Check sheet for the modelled part. Datum: model origin and axes. Units: mm. Round coordinates to 2 decimals unless told otherwise and drop trailing zeros. Order: outer loops, then holes, each group sorted by start corner. A loop starts at its lowest first (then second) coordinate and runs counter-clockwise, first axis right, second up. Notation, with made-up numbers: (12, 82) -> (61, 82) arc R13 ccw to (61, 101) -> close; hole circle Ø7 at (14, -7.5). An arc over 180 degrees is marked (long way). Answer in a Markdown table with one row per item.
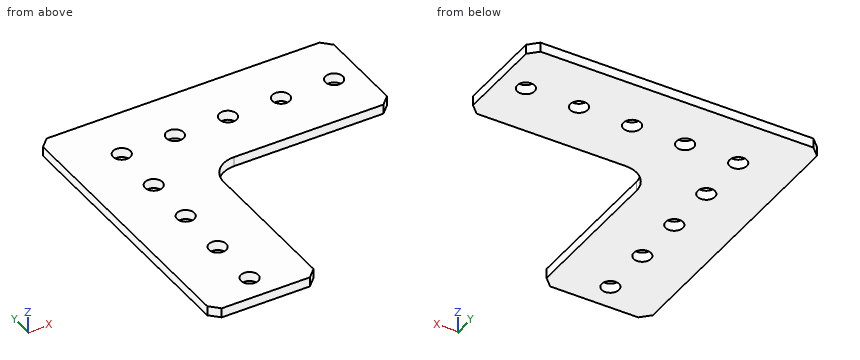
```python
from build123d import *

# Parameters (mm, degrees)
SKETCH1_R           = 2.0701
BOSS_EXTRUDE1_DEPTH = 2.286


with BuildPart() as part:
    # Sketch1 → Boss-Extrude1 (new body)
    with BuildSketch(Plane(origin=(0, 0, 0), x_dir=(-1, 0, 0), z_dir=(0, 0, -1))):
        with BuildLine():
            Line((10.414, 12.573), (-54.864, 12.573))
            Line((-54.864, 12.573), (-57.023, 10.414))
            Line((-57.023, 10.414), (-57.023, -10.668))
            Line((-57.023, -10.668), (-54.864, -12.827))
            Line((-54.864, -12.827), (-19.177, -12.827))
            ThreePointArc((-19.177, -12.827), (-14.686871939, -14.686871939), (-12.827, -19.177))
            Line((-12.827, -19.177), (-12.827, -54.864))
            Line((-12.827, -54.864), (-10.668, -57.023))
            Line((-10.668, -57.023), (10.414, -57.023))
            Line((10.414, -57.023), (12.573, -54.864))
            Line((12.573, -54.864), (12.573, 10.414))
            Line((12.573, 10.414), (10.414, 12.573))
        make_face()
        with Locations((0, -50.8)):
            Circle(SKETCH1_R, mode=Mode.SUBTRACT)
        with Locations((0, -25.4)):
            Circle(SKETCH1_R, mode=Mode.SUBTRACT)
        with Locations((-38.1, 0)):
            Circle(SKETCH1_R, mode=Mode.SUBTRACT)
        with Locations((-12.7, 0)):
            Circle(SKETCH1_R, mode=Mode.SUBTRACT)
        Circle(SKETCH1_R, mode=Mode.SUBTRACT)
        with Locations((-25.4, 0)):
            Circle(SKETCH1_R, mode=Mode.SUBTRACT)
        with Locations((0, -12.7)):
            Circle(SKETCH1_R, mode=Mode.SUBTRACT)
        with Locations((0, -38.1)):
            Circle(SKETCH1_R, mode=Mode.SUBTRACT)
        with Locations((-50.8, 0)):
            Circle(SKETCH1_R, mode=Mode.SUBTRACT)
    extrude(amount=-BOSS_EXTRUDE1_DEPTH)


solid = part.part
```
(1) Section check C-C on y = 0. Record the boundary of the cut face in (x, z), plus the area to 3 significant figures.
Solutions:
| item | result |
|---|---|
| outline | (-12.57, 0) -> (-2.07, 0) -> (-2.07, 2.29) -> (-12.57, 2.29) -> close; (2.07, 0) -> (10.63, 0) -> (10.63, 2.29) -> (2.07, 2.29) -> close; (14.77, 0) -> (23.33, 0) -> (23.33, 2.29) -> (14.77, 2.29) -> close; (27.47, 0) -> (36.03, 0) -> (36.03, 2.29) -> (27.47, 2.29) -> close; (40.17, 0) -> (48.73, 0) -> (48.73, 2.29) -> (40.17, 2.29) -> close; (52.87, 0) -> (57.02, 0) -> (57.02, 2.29) -> (52.87, 2.29) -> close |
| area | 112 mm^2 |
(2) Scan lines: probe 1 along Y at (x, z) = (0, 1.75); probe 2 along Y at (x, z) = (38.1, 1); probe 3 along X at (y, z) = (-27.5, 0.2). Record each from-to range of solid material in increasing order. Write a range as from..to.
Solutions:
| item | result |
|---|---|
| probe 1 | -57.02..-52.87, -48.73..-40.17, -36.03..-27.47, -23.33..-14.77, -10.63..-2.07, 2.07..12.57 |
| probe 2 | -12.83..-2.07, 2.07..12.57 |
| probe 3 | -12.57..12.83 |
(3) Section check A-A on x = 25.4. Record the boundary of the cut face in (y, z).
Solutions:
| item | result |
|---|---|
| outline | (-12.83, 0) -> (-2.07, 0) -> (-2.07, 2.29) -> (-12.83, 2.29) -> close; (2.07, 0) -> (12.57, 0) -> (12.57, 2.29) -> (2.07, 2.29) -> close |
(4) Depth check by flat-ended pin: pin 1 Ø1 at (x, z) = (41.5, 0.5) entering from -Y. Enter the tip coordinate at first touch or a pass-through.
Solutions:
| item | result |
|---|---|
| pin 1 | y = -12.83 |
(5) Section check B-B on x = 0. Record the boundary of the cut face in (y, z), plus the area to 3 significant figures.
Solutions:
| item | result |
|---|---|
| outline | (-57.02, 0) -> (-52.87, 0) -> (-52.87, 2.29) -> (-57.02, 2.29) -> close; (-48.73, 0) -> (-40.17, 0) -> (-40.17, 2.29) -> (-48.73, 2.29) -> close; (-36.03, 0) -> (-27.47, 0) -> (-27.47, 2.29) -> (-36.03, 2.29) -> close; (-23.33, 0) -> (-14.77, 0) -> (-14.77, 2.29) -> (-23.33, 2.29) -> close; (-10.63, 0) -> (-2.07, 0) -> (-2.07, 2.29) -> (-10.63, 2.29) -> close; (2.07, 0) -> (12.57, 0) -> (12.57, 2.29) -> (2.07, 2.29) -> close |
| area | 112 mm^2 |
(6) Section check D-D on y = -50.8. Record the boundary of the cut face in (x, z).
Solutions:
| item | result |
|---|---|
| outline | (-12.57, 0) -> (-2.07, 0) -> (-2.07, 2.29) -> (-12.57, 2.29) -> close; (2.07, 0) -> (12.83, 0) -> (12.83, 2.29) -> (2.07, 2.29) -> close |
